Here's how the part is built. I have some questions about the finished solid (model axes, mm). Face numbers are marked on the shaded views. A direction names the side the tool comes from. Round coordinates to 2 decimals unless told otherwise and drop trailing zeros. Order: outer loops, then holes, each group sorted by start corner. A loop starts at its lowest first (then second) coordinate and runs counter-clockwise, first axis right, second up. Notation, with made-up numbers: (50.25, 5) -> (82.25, 5) arc R38 ccw to (82.25, 43) -> close; hole circle Ø8 at (-39.5, 2.5). An arc over 180 degrees is marked (long way). Use a Markdown table: item, result. Add a question column.
(1) I want a section at D-D, the plane y = 79.5. Please give me the cut outline in (x, z), then the cut area to 3 significant figures.
(2) If I drill on probe 1 along X at (y, z) = (131, 6.5); probe 2 along X at (y, z) = (100.5, 8.75); probe 3 along Y at (x, z) = (-21, 2), over which ranges is the centre line in solid material (lowest first)?
(3) Thinking about a two-plate mould opening in X: for the marked faces 1, 2 and 3, which applies, pulls with the +X half, pulls with the -X half, needs draft (parallel to the pull), parting line crosses it, or undercut?
(4) I want a section at A-A, the plane y = 31. Please give me the cut outline in (x, z).
(5) I want a section at B-B, the plane x = 0. Please give me the cut outline in (y, z).
(6) On a 3-axis mill with a long thin cutter (end or side, diameter ignored), from which of +Z, -Z, +X, -X, +Y, -Y can I reach the whole of each face in a straight line? I mean the marked faces 4 and 5. Say none if no direction works.
(7) I want a section at C-C, the plane z = 7.75. Give the number of separate pieces and of enclosed holes in the cut face, then the cut area to 3 significant figures.
from build123d import *

# Parameters (mm, degrees)
SKETCH_R   = 2.15
SKETCH_R_2 = 16
PAD_DEPTH  = 10


with BuildPart() as part:
    # Sketch → Pad (new body)
    with BuildSketch(Plane.XY):
        with BuildLine():
            Line((-30.5, 141), (-30.5, -0.5))
            ThreePointArc((-30.5, -0.5), (0, -31), (30.5, -0.5))
            Line((30.5, -0.5), (30.5, 141))
            Line((30.5, 141), (-30.5, 141))
        make_face()
        with Locations((-20.5, 131)):
            Circle(SKETCH_R, mode=Mode.SUBTRACT)
        with Locations((20.5, 131)):
            Circle(SKETCH_R, mode=Mode.SUBTRACT)
        with Locations((-20.5, 96)):
            Circle(SKETCH_R, mode=Mode.SUBTRACT)
        with Locations((20.5, 96)):
            Circle(SKETCH_R, mode=Mode.SUBTRACT)
        Circle(SKETCH_R_2, mode=Mode.SUBTRACT)
        with Locations((-20.5, 31)):
            Circle(SKETCH_R, mode=Mode.SUBTRACT)
        with Locations((20.5, 31)):
            Circle(SKETCH_R, mode=Mode.SUBTRACT)
        with BuildLine():
            ThreePointArc((10, 116), (0, 126), (-10, 116))
            Line((-10, 116), (-10, 46))
            ThreePointArc((-10, 46), (0, 36), (10, 46))
            Line((10, 116), (10, 46))
        make_face(mode=Mode.SUBTRACT)
    extrude(amount=PAD_DEPTH)


solid = part.part
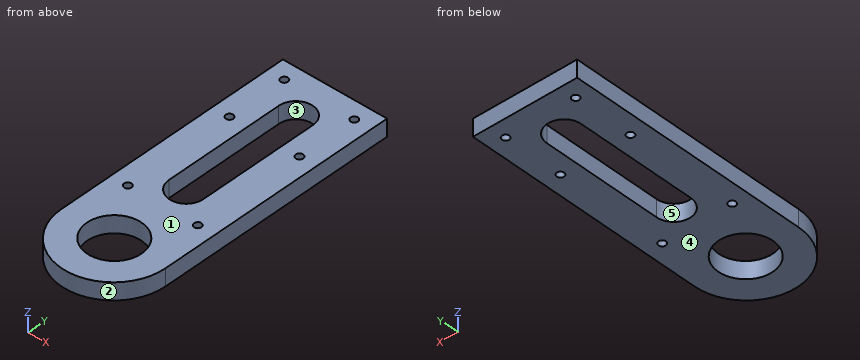
Taken from the geometry:
| question | item | result |
|---|---|---|
| 1 | outline | (-30.5, 0) -> (-10, 0) -> (-10, 10) -> (-30.5, 10) -> close; (10, 0) -> (30.5, 0) -> (30.5, 10) -> (10, 10) -> close |
| 1 | area | 410 mm2 |
| 2 | probe 1 | x = -30.5 to -22.65, -18.35 to 18.35, 22.65 to 30.5 |
| 2 | probe 2 | x = -30.5 to -10, 10 to 30.5 |
| 2 | probe 3 | y = -22.62 to 28.91, 33.09 to 93.91, 98.09 to 128.91, 133.09 to 141 |
| 3 | face 1 | needs draft |
| 3 | face 2 | parting line crosses it |
| 3 | face 3 | undercut |
| 4 | outline | (-30.5, 0) -> (-22.65, 0) -> (-22.65, 10) -> (-30.5, 10) -> close; (-18.35, 0) -> (18.35, 0) -> (18.35, 10) -> (-18.35, 10) -> close; (22.65, 0) -> (30.5, 0) -> (30.5, 10) -> (22.65, 10) -> close |
| 5 | outline | (-31, 0) -> (-16, 0) -> (-16, 10) -> (-31, 10) -> close; (16, 0) -> (36, 0) -> (36, 10) -> (16, 10) -> close; (126, 0) -> (141, 0) -> (141, 10) -> (126, 10) -> close |
| 6 | face 4 | -Z, +X, -X, +Y, -Y |
| 6 | face 5 | +Z, -Z |
| 7 | separate pieces | 1 |
| 7 | enclosed holes | 8 |
| 7 | area | 7,490 mm2 |
